Answer from the drawing. Dimensions are ordinates in mm from the lowest x, y and z of the part. Give positions to 0.01 mm unless a question says otherwise; leave off trailing zeros. Order: outer loops, then holes, each group sorted by start corner. A loop starts at its lowest first (then second) coordinate and runs counter-clockwise, first axis right, second up.
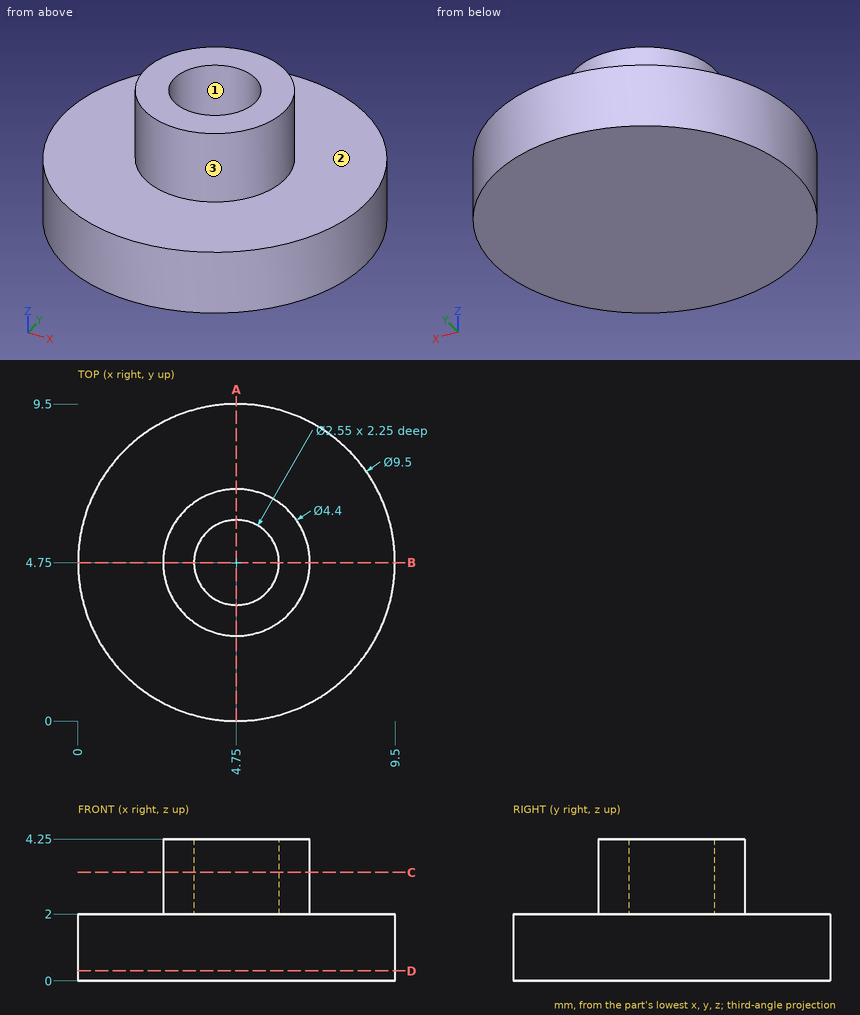
1) Consider L1, parallel to Y at x = 4.75, z = 3.1 (3 decimals); L2, parallel to Z at x = 5.75, y = 6.75; L3, parallel to X at y = 4.25, z = 2.75. Determine where each line is inside the solid, lowest interval first.
Final values:
L1: y = 2.55 to 3.475, 6.025 to 6.95
L2: z = 0 to 2
L3: x = 2.61 to 3.58, 5.92 to 6.89
2) For a pull along Y with two mould halves and no side action, classify the marked faces 1, 2 and 3 as released by +Y, released by -Y, zero draft, split by the parting line, or undercut.
Final values:
face 1: undercut
face 2: zero draft
face 3: split by the parting line
3) Given pin 1 (1.5 mm diameter, centred on x = 6.5, z = 2, fed in from +Y); pin 2 (1.5 mm diameter, centred on x = 6.5, z = 2.5, fed in from +Y), each flat-ended and moving along its own axis, determine where each tip first touches the part or whether it passes through.
Final values:
pin 1: stops at y = 9.39
pin 2: stops at y = 9.35
4) The part is cut by section C-C on z = 3.25. Determine the outline of the cut face in (x, y) (3 decimals), and give its area (3 significant figures).
Final values:
outline: circle Ø4.4 at (4.75, 4.75); hole circle Ø2.55 at (4.75, 4.75)
area: 10.1 mm2
5) The part is cut by section A-A on x = 4.75. Determine the outline of the cut face in (y, z) (3 decimals).
Final values:
outline: (0, 0) - (9.5, 0) - (9.5, 2) - (6.95, 2) - (6.95, 4.25) - (6.025, 4.25) - (6.025, 2) - (3.475, 2) - (3.475, 4.25) - (2.55, 4.25) - (2.55, 2) - (0, 2) - close
6) The part is cut by section D-D on z = 0.3. Determine the outline of the cut face in (x, y).
Final values:
outline: circle Ø9.5 at (4.75, 4.75)
